Input: part model. Units: mm. Frame: model coordinates. A direction names the side the tool comes from. Coordinates: 2 decimals unless noted, no trailing zeros. Write each loop counter-clockwise with the first axis right and the second up, starting at its lowest first coordinate (ties: lowest second). Pieces come first, ordered by that corner, then holes.
1) Section query B-B (y = -66). Output: boundary loops of the cut face in (x, z).
2) Set-up query: faces 5 (the flat face through (-200, 425, 152)), 6 (the flat face through (3, -440, 137)), 7 (the flat face through (-3, 410, 148)). Return all of +Z, -Z, +X, -X, +Y, -Y with unobstructed straight access to the full face (end or side cutting, diameter ignored); none if empty.
3) Line query: L1, parallel to Y at x = 214, z = 150; L2, parallel to Y at x = 42.5, z = 265.5; L3, parallel to X at y = 178, z = 264. Output: solid intervals per line, ascending.
4) Section query C-C (x = -92.5). Output: boundary loops of the cut face in (y, z), then the cut area to 3 significant figures.
5) Draft query along Y for faces 1 (the flat face through (3, 440, 137)), 2 (the flat face through (3, 6, -30)), 3 (the flat face through (200, -6, 148)), 4 (the flat face through (-18, 21, 0)). Return one class per face: pulls with the +Y half, pulls with the -Y half, needs draft (parallel to the pull), parting line crosses it, or undercut.
6) Section query A-A (z = 98). Output: boundary loops of the cut face in (x, y), then the cut area to 3 significant figures.
7) Pin query (flat end, axial travel): pin 1 Ø10 at (x, y) = (-88.5, -239) entering from +Z; pin 2 Ø1.5 at (y, z) = (-156, 150.5) entering from -X; pin 3 Ø15 at (y, z) = (417.5, 183.5) entering from -X. Return the tip coordinate at first contact, or that it passes through.
from build123d import *

# Parameters (mm, degrees)
SKETCH1_W           = 460
SKETCH1_H           = 880
SKETCH1_W_2         = 400
SKETCH1_H_2         = 820
BOSS_EXTRUDE1_DEPTH = 300
SKETCH2_W           = 460
SKETCH2_H           = 880
BOSS_EXTRUDE2_DEPTH = 30
SKETCH3_R           = 4
CUT_EXTRUDE1_DEPTH  = 460
SKETCH4_W           = 30
SKETCH4_H           = 850
CUT_EXTRUDE2_DEPTH  = 300


with BuildPart() as part:
    # Sketch1 → Boss-Extrude1 (new body)
    with BuildSketch(Plane.XY):
        Rectangle(SKETCH1_W, SKETCH1_H)
        Rectangle(SKETCH1_W_2, SKETCH1_H_2, mode=Mode.SUBTRACT)
    extrude(amount=BOSS_EXTRUDE1_DEPTH)

    # Sketch2 → Boss-Extrude2 (add)
    with BuildSketch(Plane(origin=(0, 0, 0), x_dir=(-1, 0, 0), z_dir=(0, 0, -1))):
        Rectangle(SKETCH2_W, SKETCH2_H)
    extrude(amount=BOSS_EXTRUDE2_DEPTH)

    # Sketch3 → Cut-Extrude1 (cut)
    with BuildSketch(Plane(origin=(230, 0, 0), x_dir=(0, 0, -1), z_dir=(1, 0, 0))):
        with Locations((-150, 190)):
            Circle(SKETCH3_R)
        with Locations((-150, 90)):
            Circle(SKETCH3_R)
        with Locations((-150, -10)):
            Circle(SKETCH3_R)
        with Locations((-150, -110)):
            Circle(SKETCH3_R)
        with Locations((-150, -210)):
            Circle(SKETCH3_R)
    extrude(amount=-CUT_EXTRUDE1_DEPTH, mode=Mode.SUBTRACT)

    # Sketch4 → Cut-Extrude2 (cut)
    with BuildSketch(Plane.XY.offset(300)):
        with Locations((-215, 15)):
            Rectangle(SKETCH4_W, SKETCH4_H)
    extrude(amount=-CUT_EXTRUDE2_DEPTH, mode=Mode.SUBTRACT)


solid = part.part
Answer:
1. outline: (-230, -30) - (230, -30) - (230, 300) - (200, 300) - (200, 0) - (-230, 0) - close
2. face 5: +Z, -X, +Y
2. face 6: +Z, -Z, +X, -X, -Y
2. face 7: +Z, -X
3. L1: y = -440 to -214, -206 to -114, -106 to -14, -6 to 86, 94 to 186, 194 to 440
3. L2: y = -440 to -410, 410 to 440
3. L3: x = 200 to 230
4. outline: (-440, -30) - (440, -30) - (440, 300) - (410, 300) - (410, 0) - (-410, 0) - (-410, 300) - (-440, 300) - close
4. area: 44,400 mm2
5. face 1: pulls with the +Y half
5. face 2: needs draft
5. face 3: undercut
5. face 4: undercut
6. outline: (-230, -440) - (230, -440) - (230, 440) - (-200, 440) - (-200, 410) - (200, 410) - (200, -410) - (-230, -410) - close
6. area: 51,300 mm2
7. pin 1: stops at z = 0
7. pin 2: stops at x = 200
7. pin 3: stops at x = -200
